For this review, use the dimensioned drawing (mm, ordinates from the lowest corner) and the shaded views. Round coordinates to 2 decimals unless told otherwise and drop trailing zeros. Order: outer loops, then holes, each group sorted by start corner. A loop starts at its lowest first (then second) coordinate and runs counter-clockwise, first axis right, second up. Notation, with made-up numbers: (-39, 9) - (-30, 9) arc R23 ccw to (-30, 26) - close; hole circle Ø10 at (71.25, 21). An arc over 180 degrees is marked (long way). Write item = value, one per line.
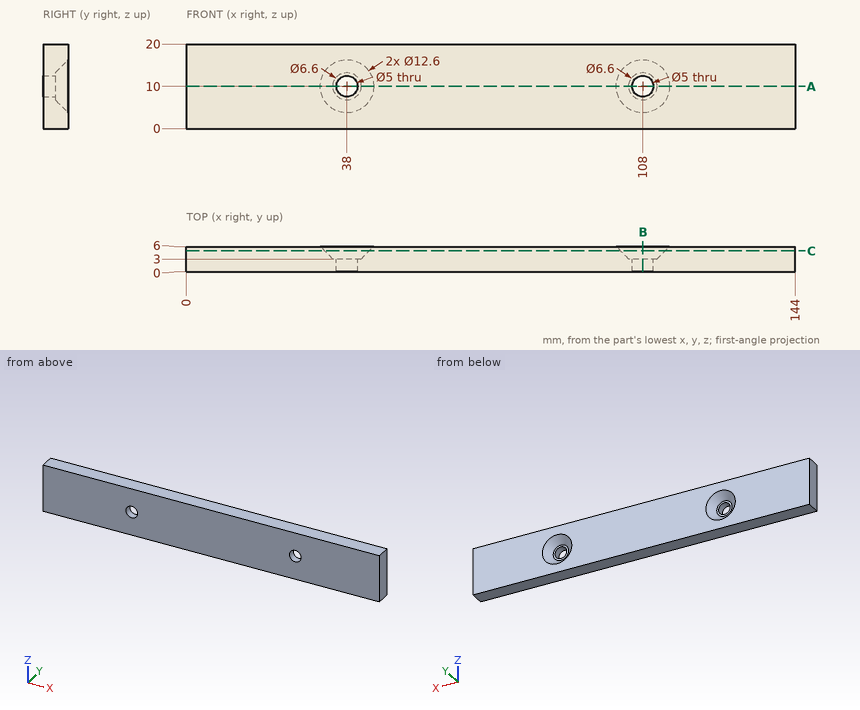
1) To check wall thickness, follow L1, parallel to X at y = 1.3, z = 10; L2, parallel to Z at x = 38, y = 1.7; L3, parallel to X at y = 5.5, z = 6.5. State the ranges of each line that lie inside material, in increasing order. Write a range as from..to.
Findings:
L1 = 0..35.5, 40.5..105.5, 110.5..144
L2 = 0..7.5, 12.5..20
L3 = 0..33.38, 42.62..103.38, 112.62..144
2) We need section C-C on y = 4.95. Write out the cut boundary in (x, z), and give its area (3 significant figures).
Findings:
outline = (0, 0) - (144, 0) - (144, 20) - (0, 20) - close; hole circle Ø10.5 at (38, 10); hole circle Ø10.5 at (108, 10)
area = 2,710 mm^2
3) We need section B-B on x = 108. Write out the cut boundary in (y, z), and give its area (3 significant figures).
Findings:
outline = (0, 0) - (6, 0) - (6, 3.7) - (3, 6.7) - (3, 7.5) - (0, 7.5) - close; (0, 12.5) - (3, 12.5) - (3, 13.3) - (6, 16.3) - (6, 20) - (0, 20) - close
area = 76.2 mm^2
4) We need section A-A on z = 10. Write out the cut boundary in (x, y).
Findings:
outline = (0, 0) - (35.5, 0) - (35.5, 3) - (34.7, 3) - (31.7, 6) - (0, 6) - close; (40.5, 0) - (105.5, 0) - (105.5, 3) - (104.7, 3) - (101.7, 6) - (44.3, 6) - (41.3, 3) - (40.5, 3) - close; (110.5, 0) - (144, 0) - (144, 6) - (114.3, 6) - (111.3, 3) - (110.5, 3) - close
5) Clearance check with a flat-ended pin moving along its axis: pin 1 Ø7.5 at (x, z) = (108.5, 10) entering from +Y. State where the tip first meets the part, or that it passes through.
Findings:
pin_1 = 3.95
